```python
from build123d import *

# Parameters (mm, degrees)
SKETCH018_W    = 135
SKETCH018_H    = 46.2
PAD008_DEPTH   = 57
THICKNESS001_T = 3
SKETCH019_R    = 10
PAD009_DEPTH   = 6
PAD010_DEPTH   = 14


with BuildPart() as part:
    # Sketch018 → Pad008 (new body)
    with BuildSketch(Plane.XZ):
        with Locations((67.5, 23.1)):
            Rectangle(SKETCH018_W, SKETCH018_H)
    extrude(amount=PAD008_DEPTH)

    # Thickness001
    thickness001_openings = [part.faces().sort_by_distance(p)[0] for p in [
        (135, -28.5, 23.1),
        (67.5, 0, 23.1),
        (0, -28.5, 23.1),
    ]]
    offset(amount=THICKNESS001_T, openings=thickness001_openings, kind=Kind.INTERSECTION)

    # Sketch019 (on Face10 of Thickness001) → Pad009 (join)
    with BuildSketch(Plane.XZ.offset(60)):
        with Locations((67.5, 23.1)):
            Circle(SKETCH019_R)
    extrude(amount=PAD009_DEPTH)

    # Sketch020 (on Face12 of Pad009) → Pad010 (join)
    with BuildSketch(Plane.XZ.offset(66)):
        Polygon((60, 36.090381), (52.5, 23.1), (60, 10.109619), (75, 10.109619), (82.5, 23.1), (75, 36.090381), align=None)
    extrude(amount=PAD010_DEPTH)


solid = part.part
```
CAD build for the part. Positions are in the model's coordinates, mm. A direction names the side the tool comes from. Coordinates: 2 decimals unless noted, no trailing zeros. Order: outer loops, then holes, each group sorted by start corner. A loop starts at its lowest first (then second) coordinate and runs counter-clockwise, first axis right, second up. Notation, with made-up numbers: (40, 12) - (71, 12) arc R15 cw to (71, 26) - close; hole circle Ø7 at (1, -34.5). An arc over 180 degrees is marked (long way). Answer in a Markdown table with one row per item.
1. Drill centre lines: L1, parallel to Y at x = 62, z = 32.5; L2, parallel to Z at x = 78.5, y = -2.5; L3, parallel to Y at x = 50, z = 3.5. Where is each one in solid material? Low to high. Write a range as from..to.
Answer:
| item | result |
|---|---|
| L1 | -80..-66, -60..-57 |
| L2 | -3..0, 46.2..49.2 |
| L3 | -60..-57 |
2. Slice it at C-C, the plane z = 4. List the corners of the cut face in (x, y).
Answer:
| item | result |
|---|---|
| outline | (0, -60) - (135, -60) - (135, -57) - (0, -57) - close |
3. Pull direction Z, two halves, no side cores. Call faces 4 (the face through (67, -57, 23)), 5 (the face through (67, -28, 0)), 6 (the face through (67, -30, 49.2)), 7 (the face through (67, 0, -1)): +Z half, -Z half, draft (parallel to the pull), parting line (faces both ways), or undercut.
Answer:
| item | result |
|---|---|
| face 4 | undercut |
| face 5 | undercut |
| face 6 | +Z half |
| face 7 | draft |
4. Slice it at B-B, the plane x = 67.5. List the corners of the cut face in (y, z).
Answer:
| item | result |
|---|---|
| outline | (-80, 10.11) - (-66, 10.11) - (-66, 13.1) - (-60, 13.1) - (-60, -3) - (0, -3) - (0, 0) - (-57, 0) - (-57, 46.2) - (0, 46.2) - (0, 49.2) - (-60, 49.2) - (-60, 33.1) - (-66, 33.1) - (-66, 36.09) - (-80, 36.09) - close |
5. Slice it at D-D, the plane x = 23.5. List the corners of the cut face in (y, z).
Answer:
| item | result |
|---|---|
| outline | (-60, -3) - (0, -3) - (0, 0) - (-57, 0) - (-57, 46.2) - (0, 46.2) - (0, 49.2) - (-60, 49.2) - close |
6. Slice it at A-A, the plane y = -43. List the corners of the cut face in (x, z).
Answer:
| item | result |
|---|---|
| outline | (0, -3) - (135, -3) - (135, 0) - (0, 0) - close; (0, 46.2) - (135, 46.2) - (135, 49.2) - (0, 49.2) - close |
7. 3-axis set-ups, long thin cutter, end or side, ignore diameter. For faces 1 (the face through (68, -73, 36.09)), 2 (the face through (74, -66, 15)), 3 (the face through (78.698, -72.902, 16.514)): which of +Z, -Z, +X, -X, +Y, -Y reach the whole face in a straight line?
Answer:
| item | result |
|---|---|
| face 1 | +Z, +X, -X, -Y |
| face 2 | none |
| face 3 | -Z, +X, -Y |
8. Flat gauge pins, fed straight in: P1, Ø14, axis at x = 73, z = 12.5, coming from the +Y side; P2, Ø15.5, axis at x = 65, y = -69.5, coming from the -Z side; P3, Ø11, axis at x = 66.5, y = -72, coming from the +Z side. Where does each tip first touch, or does it go through?
Answer:
| item | result |
|---|---|
| P1 | y = -57 |
| P2 | z = 10.11 |
| P3 | z = 36.09 |
